For this review, take the finished solid that the model builds, in its own axes (mm). Face numbers are marked on the shaded views. Give positions to 0.01 mm unless a question says otherwise; leave off trailing zeros. Loops run counter-clockwise (first coordinate to the right, second up) from the corner with the lowest first, then second, coordinate; pieces in that order, holes last. Notation, with made-up numbers: M -17,39.25 L 21,39.25 A11 cw 21,59.25 Z; hole C -27.5,46.25 d6. An arc over 180 degrees is marked long. Use CSV: the item, a comma, the result in double quotes. Start each with the question number.
1. Take a section at C-C, the plane y = 12. Write out the cut boundary in (x, z), and give its area (3 significant figures).
2. Take a section at A-A, the plane z = 3.5. State how many separate pieces and enclosed holes the cut face has, and give its area (3 significant figures).
3. The part is to be moulded in two halves that separate along X. For the marked faces 1 and 2, say which applies: pulls with the +X half, pulls with the -X half, needs draft (parallel to the pull), parting line crosses it, or undercut.
4. Take a section at B-B, the plane x = 23. Write out the cut boundary in (y, z), and give its area (3 significant figures).
5. Insertion check: P1, Ø10, axis at y = -10.5, z = 8, coming from the +X side; P2, Ø1, axis at y = -9, z = 1.5, coming from the +X side; P3, Ø10, axis at x = 26, z = 17.5, coming from the +Y side. Each pin has a flat end and moves straight along its axis. Give the tip position at first contact, or say it passes through.
6. To check wall thickness, follow line 1 (Y direction, x = 30, z = 14.75); line 2 (X direction, y = 24.5, z = 20.5); line 3 (X direction, y = 25, z = 10.25). State the ranges of each line that lie inside material, in increasing order. Write a range as [from, to].
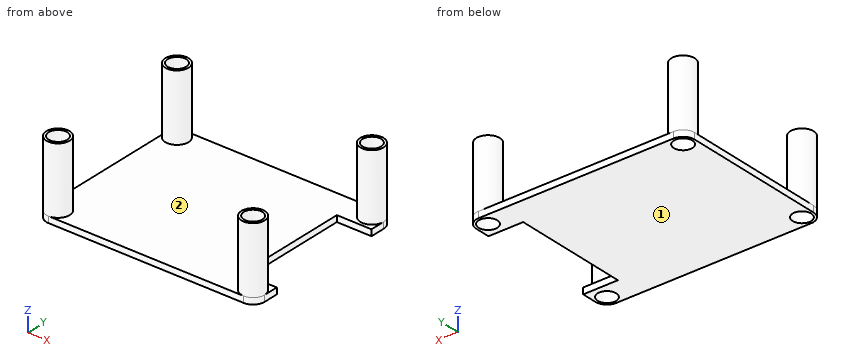
from build123d import *

# Parameters (mm, degrees)
F1_DEPTH = 2
F2_R     = 3.75
F3_DEPTH = 21.415625
F4_R     = 2.975
F5_DEPTH = 23.416625
F7_DEPTH = 2.001


with BuildPart() as f1:
    # F0 (on Top) → F1 (new body)
    with BuildSketch(Plane.XY):
        with BuildLine():
            Line((-31.3531, -27.1655), (31.3531, -27.1655))
            ThreePointArc((31.3531, -27.1655), (34.00475, -26.06715), (35.1031, -23.4155))
            Line((35.1031, -23.4155), (35.1031, 23.4155))
            ThreePointArc((35.1031, 23.4155), (34.00475, 26.06715), (31.3531, 27.1655))
            Line((31.3531, 27.1655), (-31.3531, 27.1655))
            ThreePointArc((-31.3531, 27.1655), (-34.00475, 26.06715), (-35.1031, 23.4155))
            Line((-35.1031, 23.4155), (-35.1031, -23.4155))
            ThreePointArc((-35.1031, -23.4155), (-34.00475, -26.06715), (-31.3531, -27.1655))
        make_face()
    extrude(amount=F1_DEPTH)

    # F2 (on face) → F3 (join)
    with BuildSketch(Plane.XY.offset(2)):
        with Locations((-31.3531, 23.4155)):
            Circle(F2_R)
        with Locations((31.3531, 23.4155)):
            Circle(F2_R)
        with Locations((-31.3531, -23.4155)):
            Circle(F2_R)
        with Locations((31.3531, -23.4155)):
            Circle(F2_R)
    extrude(amount=F3_DEPTH)

    # F4 (on face) → F5 (cut, through all)
    with BuildSketch(Plane.XY.offset(23.415625)):
        with Locations((-31.3531, 23.4155)):
            Circle(F4_R)
        with Locations((31.3531, 23.4155)):
            Circle(F4_R)
        with Locations((31.3531, -23.4155)):
            Circle(F4_R)
        with Locations((-31.3531, -23.4155)):
            Circle(F4_R)
    extrude(amount=-F5_DEPTH, mode=Mode.SUBTRACT)

    # F6 (on face) → F7 (cut, through all)
    with BuildSketch(Plane.XY.offset(2)):
        Polygon((23.9531, 18.653), (23.9531, 0), (23.9531, -18.653), (35.1031, -18.653), (35.1031, 18.653), align=None)
    extrude(amount=-F7_DEPTH, mode=Mode.SUBTRACT)


solid = f1.part
Result set:
1,outline,"M -35.1,0 L 23.95,0 L 23.95,2 L -35.1,2 Z"
1,area,"118 mm2"
2,separate pieces,"4"
2,enclosed holes,"4"
2,area,"65.5 mm2"
3,face 1,"needs draft"
3,face 2,"undercut"
4,outline,"M -27.17,0 L 27.17,0 L 27.17,2 L -27.17,2 Z"
4,area,"109 mm2"
5,P1,"through"
5,P2,"x = 23.95"
5,P3,"y = 27.15"
6,line 1,"[-26.91, -26.06], [-20.77, -19.92], [19.92, 20.77], [26.06, 26.91]"
6,line 2,"[-34.94, -34.12], [-28.58, -27.76], [27.76, 28.58], [34.12, 34.94]"
6,line 3,"[-34.75, -33.87], [-28.84, -27.95], [27.95, 28.84], [33.87, 34.75]"
